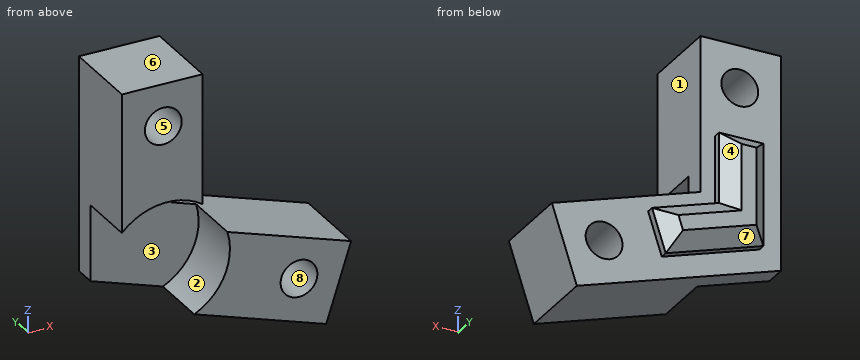
Autodesk Inventor part; units mm, degrees
ref_plane "YZ Plane" through (0, 0, 0) normal (1, 0, 0) x (0, 1, 0)
ref_plane "XZ Plane" through (0, 0, 0) normal (0, 1, 0) x (-1, 0, 0)
ref_plane "XY Plane" through (0, 0, 0) normal (0, 0, 1) x (1, 0, 0)
sketch "草图1" plane through (0, 0, 0) normal (0, 1, 0) x (-1, 0, 0)
  circle A0 centre (-11.3094, -1.4762) radius 1.25
  circle A1 centre (-2.0908, 11.2121) radius 1.25
  line L0 (-5.7974, 4.2121) -> (1.6092, -1.1691) construction
  line L1 (0.7195, 14.068) -> (0.7195, -0.5227)
  line L2 (-4.7634, 3.4608) -> (-4.7634, 14.068)
  line L3 (-4.7634, 14.068) -> (0.7195, 14.068)
  line L4 (-4.7634, 3.4608) -> (-14.8514, 0.183)
  line L5 (-14.8514, 0.183) -> (-13.1571, -5.0315)
  line L6 (-13.1571, -5.0315) -> (0.7195, -0.5227)
  point P0 (0, 0)
  dimension "d0" = 2.5
extrude "拉伸1" add sketch "草图1" along normal blind 5.5
sketch "草图3" plane through (0, 0, 0) normal (0, -1, 0) x (1, 0, 0)
  line L0 (-0.7195, -0.5227) -> (-0.7195, 14.068) construction
  line L1 (4.7634, 14.068) -> (4.7634, 3.4608) construction
  line L2 (-0.7195, -0.5227) -> (4.7634, 3.4608) construction
  circle A0 centre (2.0908, 11.2121) radius 1.25 construction
  circle A1 centre (11.3094, -1.4762) radius 1.25 construction
  line L3 (-0.7195, -0.5227) -> (-0.7195, 14.068) construction
  line L4 (13.1571, -5.0315) -> (-0.7195, -0.5227) construction
  line L5 (14.8514, 0.183) -> (13.1571, -5.0315) construction
  line L6 (4.7634, 3.4608) -> (14.8514, 0.183) construction
  line L7 (4.7634, 14.068) -> (4.7634, 3.4608) construction
  line L8 (-0.7195, 14.068) -> (4.7634, 14.068) construction
  circle A2 centre (2.3678, 1.7203) radius 4.25
  point P0 (0, 0)
  dimension "d7" = 8.5
extrude "拉伸2" cut sketch "草图3" against normal blind 4
sketch "草图5" plane through (0, 5.5, 0) normal (0, 1, 0) x (1, 0, 0)
  line L0 (-0.7195, 0.5227) -> (4.7634, -3.4608)
  line L1 (0.7578, -0.5506) -> (0.7578, -7.5215)
  line L2 (0.7578, -7.5215) -> (3.7578, -7.5215)
  line L3 (3.7578, -7.5215) -> (3.7578, -2.7302)
  line L4 (0.7578, -0.5506) -> (7.3875, 1.6036)
  line L5 (7.3875, 1.6036) -> (8.3146, -1.2496)
  line L6 (8.3146, -1.2496) -> (3.7578, -2.7302)
  circle A0 centre (2.0908, -11.2121) radius 1.25 construction
  point P0 (0, 0)
  dimension "d15" = 7.3812
extrude "拉伸3" add sketch "草图5" along normal blind 1.5
chamfer "倒角1" distance 1 angle 45 6 edges at (2.2578, 7, 7.5215) (3.7578, 7, 5.1258) (6.0362, 7, 1.9899) (7.851, 7, -0.177) (4.0727, 7, -0.5265) (0.7578, 7, 4.036)
sketch "草图6" plane through (0, 5.5, 0) normal (0, 1, 0) x (1, 0, 0)
  point P0 (0, 0)
properties part number "鸦片下"
Can you work these out from the model? Positions are in its coordinate system, mm. Face numbers are marked on the shaded views. A direction names the side the tool comes from. Give positions to 0.01 mm unless a question says otherwise; leave off trailing zeros. Order: outer loops, then holes, each group sorted by start corner. A loop starts at its lowest first (then second) coordinate and runs counter-clockwise, first axis right, second up. Notation, with made-up numbers: M 47,3.25 L 60,3.25 A23 cw 60,19.25 Z; hole C 74,45.25 d7. An arc over 180 degrees is marked long. One line per item, written item: value.
Item 1: For the marked faces 1, 2, 3 and 4, which set-ups out of +Z, -Z, +X, -X, +Y, -Y let a thin tool reach every point of the face, with its end or its side?
Verdict:
face 1: +Z, +X, +Y, -Y
face 2: -X, -Y
face 3: -Y
face 4: +Z, +X, +Y
Item 2: For pin 1 (3 mm diameter, centred on y = 4.5, z = 6, fed in from +X); pin 2 (4 mm diameter, centred on x = 10.5, y = 1.5, fed in from -Z); pin 3 (1.5 mm diameter, centred on x = 7, y = 4.5, fed in from +Z); pin 4 (4 mm diameter, centred on x = 2.09, z = 11.21, fed in from -Y), each with a flat end and sliding along its axis, tell me the tip position at first contact or that it passes through.
Verdict:
pin 1: x = 4.76
pin 2: z = -4.82
pin 3: z = 2.98
pin 4: y = 0
Item 3: If we section it at B-B on z = 12: Write out the boundary of the cut face in (x, y), and give its area (3 significant figures).
Verdict:
outline: M -0.72,0 L 1.12,0 L 1.12,5.5 L -0.72,5.5 Z; M 3.06,0 L 4.76,0 L 4.76,5.5 L 3.06,5.5 Z
area: 19.5 mm2
Item 4: If we mould it in two halves opening along X, with no side actions, what happens to the marked faces 5, 6, 7 and 8? For each: pulls with the +X half, pulls with the -X half, needs draft (parallel to the pull), parting line crosses it, or undercut.
Verdict:
face 5: undercut
face 6: needs draft
face 7: pulls with the -X half
face 8: undercut
Item 5: If we section it at C-C on x = 1.5: Write out the boundary of the cut face in (y, z), and give its area (3 significant figures).
Verdict:
outline: M 0,5.88 L 4,5.88 L 4,-1.24 L 5.5,-1.24 L 5.5,0.31 L 6,0.31 L 6.74,1.09 L 6.74,6.78 L 6,7.52 L 5.5,7.52 L 5.5,10.11 L 0,10.11 Z; M 0,12.31 L 5.5,12.31 L 5.5,14.07 L 0,14.07 Z
area: 52.0 mm2
Item 6: If we section it at A-A on y = 3: Write out the boundary of the cut face in (x, z), and give its area (3 significant figures).
Verdict:
outline: M -0.72,4.64 A4.25 cw 4.76,5.23 L 4.76,14.07 L -0.72,14.07 Z; M 4.19,-2.12 L 13.16,-5.03 L 14.85,0.18 L 6.45,2.91 A4.25 cw Z; hole C 2.09,11.21 d2.5; hole C 11.31,-1.48 d2.5
area: 82.7 mm2
Item 7: If we section it at D-D on z = 4: Write out the boundary of the cut face in (x, y).
Verdict:
outline: M -0.72,4 L 4.76,4 L 4.76,5.5 L 3.76,5.5 L 3.76,6 L 2.76,7 L 1.76,7 L 0.76,6 L 0.76,5.5 L -0.72,5.5 Z
Item 8: Please list where these lines run through material, in increasing order: line 1 (X direction, y = 1.5, z = 12.5); line 2 (Z direction, x = 3, y = 4.25); line 3 (X direction, y = 3.75, z = -1.75).
Verdict:
line 1: -0.72 to 4.76
line 2: -1.73 to 10.35, 12.07 to 14.07
line 3: 4.82 to 10.09, 12.53 to 14.22
